Geometry check sheet. Reference: the model listing, model coordinates, mm. Give positions to 0.01 mm unless a question says otherwise; leave off trailing zeros. Loops run counter-clockwise (first coordinate to the right, second up) from the corner with the lowest first, then second, coordinate; pieces in that order, holes last. Notation, with made-up numbers: (29, -33) -> (47, -33) arc R10 ccw to (47, -28) -> close; hole circle Ø5 at (23.25, 85). An arc over 180 degrees is marked (long way). Answer in a Markdown table with one row per item. Add a question column.
Autodesk Inventor part; units mm, degrees
ref_plane "YZ Plane" through (0, 0, 0) normal (1, 0, 0) x (0, 1, 0)
ref_plane "XZ Plane" through (0, 0, 0) normal (0, 1, 0) x (-1, 0, 0)
ref_plane "XY Plane" through (0, 0, 0) normal (0, 0, 1) x (1, 0, 0)
sketch "Sketch1" plane through (0, 0, 0) normal (0, 1, 0) x (-1, 0, 0)
  circle A0 centre (0, 0) radius 73.025
  circle A1 centre (0, 0) radius 84.1375
  line L0 (0, 0) -> (0, 84.1375) construction
  circle A2 centre (0, 65.0875) radius 1.7526
  circle A3 centre (0, 65.0875) radius 7.9375 construction
  circle A4 centre (-61.9019, 20.1131) radius 1.7526
  circle A5 centre (-61.9019, 20.1131) radius 7.9375 construction
  circle A6 centre (-38.2575, -52.6569) radius 1.7526
  circle A7 centre (-38.2575, -52.6569) radius 7.9375 construction
  circle A8 centre (38.2575, -52.6569) radius 1.7526
  circle A9 centre (38.2575, -52.6569) radius 7.9375 construction
  circle A10 centre (61.9019, 20.1131) radius 1.7526
  circle A11 centre (61.9019, 20.1131) radius 7.9375 construction
  arc A12 (-29.3651, -56.0703) -> (-44.2517, -45.2546) centre (-38.2575, -52.6569) ccw
  line L1 (-29.3651, -56.0703) -> (-32.8726, -65.2077)
  line L2 (-44.2517, -45.2546) -> (-51.858, -51.414)
  arc A13 (44.2517, -45.2546) -> (29.3651, -56.0703) centre (38.2575, -52.6569) ccw
  line L3 (29.3651, -56.0703) -> (32.8726, -65.2077)
  line L4 (44.2517, -45.2546) -> (51.858, -51.414)
  arc A14 (-5.2592, 57.1461) -> (5.2592, 57.1461) centre (0, 65.0875) ccw
  arc A15 (55.1667, 26.8483) -> (61.9019, 10.5881) centre (61.9019, 20.1131) ccw
  line L5 (61.9019, 10.5881) -> (72.2533, 10.5881)
  line L6 (0, 0) -> (61.9019, 20.1131) construction
  line L7 (55.1667, 26.8483) -> (63.8164, 35.4981)
  arc A16 (-61.9019, 10.5881) -> (-55.1667, 26.8483) centre (-61.9019, 20.1131) ccw
  line L8 (-61.9019, 10.5881) -> (-72.2533, 10.5881)
  line L9 (-55.1667, 26.8483) -> (-63.8164, 35.4981)
  line L10 (0, 0) -> (12.6807, 71.9156) construction
  circle A17 centre (11.8537, 67.2254) radius 3.3655
  circle A18 centre (0, 0) radius 68.2625 construction
  circle A19 centre (11.8537, 67.2254) radius 4.7625 construction
  circle A20 centre (-11.8537, 67.2254) radius 3.3655
  circle A21 centre (-11.8537, 67.2254) radius 4.7625 construction
  line L11 (-5.2592, 57.1461) -> (-23.4145, 69.1694)
  line L12 (5.2592, 57.1461) -> (23.4145, 69.1694)
  line L13 (7.9375, -79.375) -> (-7.9375, -79.375)
  line L14 (-7.9375, -79.375) -> (-7.9375, -73.025)
  line L15 (-7.9375, -73.025) -> (7.9375, -73.025)
  line L16 (7.9375, -73.025) -> (7.9375, -79.375)
  line L17 (7.9375, -79.375) -> (-7.9375, -73.025) construction
  line L18 (-7.9375, -79.375) -> (7.9375, -73.025) construction
  line L19 (0, -76.2) -> (0, -84.1375) construction
  line L20 (12.7, -82.55) -> (-12.7, -82.55) construction
  line L21 (-12.7, -82.55) -> (-12.7, -69.85)
  line L22 (-12.7, -69.85) -> (12.7, -69.85)
  line L23 (12.7, -69.85) -> (12.7, -82.55)
  line L24 (12.7, -82.55) -> (-12.7, -69.85) construction
  line L25 (-12.7, -82.55) -> (12.7, -69.85) construction
  line L26 (30.7823, -63.9747) -> (51.3313, -49.045)
  line L27 (36.5014, -63.744) -> (49.3446, -54.4129)
  line L28 (53.077, -59.5502) -> (40.2339, -68.8813)
  line L29 (40.2339, -68.8813) -> (36.5014, -63.744)
  line L30 (49.3446, -54.4129) -> (53.077, -59.5502)
  line L31 (53.077, -59.5502) -> (36.5014, -63.744) construction
  line L32 (40.2339, -68.8813) -> (49.3446, -54.4129) construction
  line L33 (51.3313, -49.045) -> (58.7962, -59.3195)
  line L34 (58.7962, -59.3195) -> (38.2472, -74.2492) construction
  line L35 (38.2472, -74.2492) -> (51.3313, -49.045) construction
  line L36 (58.7962, -59.3195) -> (30.7823, -63.9747) construction
  line L37 (38.2472, -74.2492) -> (30.7823, -63.9747)
  line L38 (62.5068, -33.6633) -> (70.3558, -9.5064)
  line L39 (66.9981, -30.115) -> (71.9037, -15.017)
  line L40 (77.9429, -16.9792) -> (73.0373, -32.0772)
  line L41 (73.0373, -32.0772) -> (66.9981, -30.115)
  line L42 (71.9037, -15.017) -> (77.9429, -16.9792)
  line L43 (77.9429, -16.9792) -> (66.9981, -30.115) construction
  line L44 (73.0373, -32.0772) -> (71.9037, -15.017) construction
  line L45 (70.3558, -9.5064) -> (82.4342, -13.4309)
  line L46 (82.4342, -13.4309) -> (74.5852, -37.5878) construction
  line L47 (74.5852, -37.5878) -> (70.3558, -9.5064) construction
  line L48 (82.4342, -13.4309) -> (62.5068, -33.6633) construction
  line L49 (74.5852, -37.5878) -> (62.5068, -33.6633)
  line L50 (70.3558, 9.5064) -> (62.5068, 33.6633)
  line L51 (71.9037, 15.017) -> (66.9981, 30.115)
  line L52 (73.0373, 32.0772) -> (77.9429, 16.9792)
  line L53 (77.9429, 16.9792) -> (71.9037, 15.017)
  line L54 (66.9981, 30.115) -> (73.0373, 32.0772)
  line L55 (73.0373, 32.0772) -> (71.9037, 15.017) construction
  line L56 (77.9429, 16.9792) -> (66.9981, 30.115) construction
  line L57 (62.5068, 33.6633) -> (74.5852, 37.5878)
  line L58 (74.5852, 37.5878) -> (82.4342, 13.4309) construction
  line L59 (82.4342, 13.4309) -> (62.5068, 33.6633) construction
  line L60 (74.5852, 37.5878) -> (70.3558, 9.5064) construction
  line L61 (82.4342, 13.4309) -> (70.3558, 9.5064)
  line L62 (51.3313, 49.045) -> (30.7823, 63.9747)
  line L63 (49.3446, 54.4129) -> (36.5014, 63.744)
  line L64 (40.2339, 68.8813) -> (53.077, 59.5502)
  line L65 (53.077, 59.5502) -> (49.3446, 54.4129)
  line L66 (36.5014, 63.744) -> (40.2339, 68.8813)
  line L67 (40.2339, 68.8813) -> (49.3446, 54.4129) construction
  line L68 (53.077, 59.5502) -> (36.5014, 63.744) construction
  line L69 (30.7823, 63.9747) -> (38.2472, 74.2492)
  line L70 (38.2472, 74.2492) -> (58.7962, 59.3195) construction
  line L71 (58.7962, 59.3195) -> (30.7823, 63.9747) construction
  line L72 (38.2472, 74.2492) -> (51.3313, 49.045) construction
  line L73 (58.7962, 59.3195) -> (51.3313, 49.045)
  circle A22 centre (0, 0) radius 69.85
  line L74 (17.6671, 70.8557) -> (16.0268, 64.2769)
  line L75 (-17.6671, 70.8557) -> (-16.0268, 64.2769)
  line L76 (-38.2575, -52.6569) -> (-49.4548, -68.0687) construction
  line L77 (12.7, 69.85) -> (-12.7, 69.85)
  line L78 (7.9375, 73.025) -> (-7.9375, 73.025)
  line L79 (-7.9375, 79.375) -> (7.9375, 79.375)
  line L80 (7.9375, 79.375) -> (7.9375, 73.025)
  line L81 (-7.9375, 73.025) -> (-7.9375, 79.375)
  line L82 (-7.9375, 79.375) -> (7.9375, 73.025) construction
  line L83 (7.9375, 79.375) -> (-7.9375, 73.025) construction
  line L84 (-12.7, 69.85) -> (-12.7, 82.55)
  line L85 (-12.7, 82.55) -> (12.7, 82.55) construction
  line L86 (12.7, 82.55) -> (-12.7, 69.85) construction
  line L87 (-12.7, 82.55) -> (12.7, 69.85) construction
  line L88 (12.7, 82.55) -> (12.7, 69.85)
  line L89 (-30.7823, 63.9747) -> (-51.3313, 49.045)
  line L90 (-36.5014, 63.744) -> (-49.3446, 54.4129)
  line L91 (-53.077, 59.5502) -> (-40.2339, 68.8813)
  line L92 (-40.2339, 68.8813) -> (-36.5014, 63.744)
  line L93 (-49.3446, 54.4129) -> (-53.077, 59.5502)
  line L94 (-53.077, 59.5502) -> (-36.5014, 63.744) construction
  line L95 (-40.2339, 68.8813) -> (-49.3446, 54.4129) construction
  line L96 (-51.3313, 49.045) -> (-58.7962, 59.3195)
  line L97 (-58.7962, 59.3195) -> (-38.2472, 74.2492) construction
  line L98 (-38.2472, 74.2492) -> (-51.3313, 49.045) construction
  line L99 (-58.7962, 59.3195) -> (-30.7823, 63.9747) construction
  line L100 (-38.2472, 74.2492) -> (-30.7823, 63.9747)
  line L101 (-62.5068, 33.6633) -> (-70.3558, 9.5064)
  line L102 (-66.9981, 30.115) -> (-71.9037, 15.017)
  line L103 (-77.9429, 16.9792) -> (-73.0373, 32.0772)
  line L104 (-73.0373, 32.0772) -> (-66.9981, 30.115)
  line L105 (-71.9037, 15.017) -> (-77.9429, 16.9792)
  line L106 (-77.9429, 16.9792) -> (-66.9981, 30.115) construction
  line L107 (-73.0373, 32.0772) -> (-71.9037, 15.017) construction
  line L108 (-70.3558, 9.5064) -> (-82.4342, 13.4309)
  line L109 (-82.4342, 13.4309) -> (-74.5852, 37.5878) construction
  line L110 (-74.5852, 37.5878) -> (-70.3558, 9.5064) construction
  line L111 (-82.4342, 13.4309) -> (-62.5068, 33.6633) construction
  line L112 (-74.5852, 37.5878) -> (-62.5068, 33.6633)
  line L113 (-70.3558, -9.5064) -> (-62.5068, -33.6633)
  line L114 (-71.9037, -15.017) -> (-66.9981, -30.115)
  line L115 (-73.0373, -32.0772) -> (-77.9429, -16.9792)
  line L116 (-77.9429, -16.9792) -> (-71.9037, -15.017)
  line L117 (-66.9981, -30.115) -> (-73.0373, -32.0772)
  line L118 (-73.0373, -32.0772) -> (-71.9037, -15.017) construction
  line L119 (-77.9429, -16.9792) -> (-66.9981, -30.115) construction
  line L120 (-62.5068, -33.6633) -> (-74.5852, -37.5878)
  line L121 (-74.5852, -37.5878) -> (-82.4342, -13.4309) construction
  line L122 (-82.4342, -13.4309) -> (-62.5068, -33.6633) construction
  line L123 (-74.5852, -37.5878) -> (-70.3558, -9.5064) construction
  line L124 (-82.4342, -13.4309) -> (-70.3558, -9.5064)
  line L125 (-51.3313, -49.045) -> (-30.7823, -63.9747)
  line L126 (-49.3446, -54.4129) -> (-36.5014, -63.744)
  line L127 (-40.2339, -68.8813) -> (-53.077, -59.5502)
  line L128 (-53.077, -59.5502) -> (-49.3446, -54.4129)
  line L129 (-36.5014, -63.744) -> (-40.2339, -68.8813)
  line L130 (-40.2339, -68.8813) -> (-49.3446, -54.4129) construction
  line L131 (-53.077, -59.5502) -> (-36.5014, -63.744) construction
  line L132 (-30.7823, -63.9747) -> (-38.2472, -74.2492)
  line L133 (-38.2472, -74.2492) -> (-58.7962, -59.3195) construction
  line L134 (-58.7962, -59.3195) -> (-30.7823, -63.9747) construction
  line L135 (-38.2472, -74.2492) -> (-51.3313, -49.045) construction
  line L136 (-58.7962, -59.3195) -> (-51.3313, -49.045)
  line L137 (7.633, 69.4317) -> (8.401, 59.2267)
  line L138 (-7.633, 69.4317) -> (-8.401, 59.2267)
  point P0 (51.858, -51.414)
  point P1 (64.5887, 34.0727)
  point P2 (44.7892, -61.6471)
  point P3 (72.4705, -23.5471)
  point P4 (72.4705, 23.5471)
  point P5 (44.7892, 61.6471)
  point P6 (12.7, -71.9122)
  point P7 (-12.7, -71.9122)
  point P8 (31.9944, 65.643)
  point P9 (52.5434, 50.7133)
  point P10 (64.468, 34.3005)
  point P11 (72.3171, 10.1437)
  point P12 (72.3171, -10.1437)
  point P13 (64.468, -34.3005)
  point P14 (52.5434, -50.7133)
  point P15 (31.9944, -65.643)
  point P16 (66.4313, 21.5848)
  point P17 (-20.018, 66.9201)
  point P18 (-61.4776, 33.1592)
  point P19 (20.018, 66.9201)
  point P20 (66.4313, -21.5848)
  point P21 (61.4776, 33.1592)
  point P22 (41.0568, -56.5098)
  point P23 (69.0428, 10.5881)
  point P24 (49.3775, -49.4053)
  point P25 (41.0568, 56.5098)
  point P26 (-69.0428, 10.5881)
  point P27 (-49.3775, -49.4053)
  point P28 (31.7288, -62.2279)
  point P29 (0, -69.85)
  point P30 (-31.7288, -62.2279)
  point P31 (0, 76.2)
  point P32 (-44.7892, 61.6471)
  point P33 (-72.4705, 23.5471)
  point P34 (-72.4705, -23.5471)
  point P35 (-44.7892, -61.6471)
  point P36 (32.0467, -63.0561)
  point P37 (50.0669, -49.9636)
  point P38 (70.0043, 10.5881)
  point P39 (62.7968, 32.7708)
  point P40 (12.7, 71.9122)
  point P41 (12.7, 70.4828)
  point P42 (9.1625, 69.2464)
  point P43 (-9.1625, 69.2464)
  point P44 (-12.7, 70.4828)
  point P45 (-12.7, 71.9122)
  point P46 (16.899, 67.775)
  point P47 (15.0737, 68.2041)
  point P48 (-15.0737, 68.2041)
  point P49 (-16.899, 67.775)
  dimension "d1" = 146.05
  dimension "d13" = 136.525
  dimension "d14" = 9.525
  dimension "d78" = 3.175
  dimension "d0" = 11.1125
  dimension "d2" = 3.5052
  dimension "d3" = 15.875
  dimension "d6" = 360
  dimension "d8" = 19.05
  dimension "d9" = 19.05
  dimension "d10" = 19.05
  dimension "d11" = 10
  dimension "d12" = 6.731
  dimension "d34" = 15.875
  dimension "d35" = 6.35
  dimension "d37" = 25.4
  dimension "d39" = 3.175
  dimension "d42" = 360
  dimension "d151" = 76.2
  dimension "d153" = 15
  dimension "d163" = 90
extrude "Extrusion1" add sketch "Sketch1" along normal blind 9.525 contours L12 A14 L11 L138 A22 L137
fillet "Fillet14" radius 3.175 4 edges at (-7.633, 4.7625, 69.4317) (-8.401, 4.7625, 59.2267) (8.401, 4.7625, 59.2267) (7.633, 4.7625, 69.4317)
chamfer "Chamfer15" distance 3.175 angle 45 1 edges at (1.7526, 9.525, 65.0875)
equation "\"d1\" = Ring_ID"
equation "\"BearingTol\" = 0.1"
equation "\"CSDepth\" = 1.7272"
equation "\"CSAngle\" = 41deg"
properties part number "Retaining Ring" material "UHMW, White"
1. Sectioned sample at C-C (x = 5.75). Enter the section's corners in (y, z) (3 decimals), plus the area to 3 significant figures.
2. Material ranges on L1, parallel to Z at x = 0, y = 1.75; L2, parallel to Z at x = 0.5, y = 8.75; L3, parallel to X at y = 4, z = 66.5, recorded low to high. Write a range as from..to.
3. Release check for a two-part mould opening along Z. For faces 1 (the face through (0.254, 6.549, 67.022)), 2 (the face through (0, 0, 63)), 3 (the face through (-6.043, 4.696, 57.665)) record: released by +Z, released by -Z, zero draft, split by the parting line, or undercut.
4. Sectioned sample at D-D (x = -5.5). Enter the section's corners in (y, z) (3 decimals), plus the area to 3 significant figures.
5. Sectioned sample at A-A (x = 0). Enter the section's corners in (y, z) (3 decimals).
6. Gauge pin test, flat ends, axial feed: pin 1 Ø1 at (x, y) = (-6, 5.5) entering from -Z; pin 2 Ø2 at (x, y) = (-3, 4) entering from -Z; pin 3 Ø1.5 at (x, z) = (3, 66.5) entering from +Y. Record the tip position at first contact, or that the pin passes through.
Response:
| question | item | result |
|---|---|---|
| 1 | outline | (0, 57.471) -> (9.525, 57.471) -> (9.525, 69.497) -> (0, 69.497) -> close |
| 1 | area | 115 mm2 |
| 2 | L1 | z = 55.56..63.33, 66.84..69.85 |
| 2 | L2 | z = 55.58..60.97, 69.21..69.85 |
| 2 | L3 | x = -7.85..-1.04, 1.04..7.85 |
| 3 | face 1 | undercut |
| 3 | face 2 | zero draft |
| 3 | face 3 | released by -Z |
| 4 | outline | (0, 57.306) -> (9.525, 57.306) -> (9.525, 69.576) -> (0, 69.576) -> close |
| 4 | area | 117 mm2 |
| 5 | outline | (0, 55.563) -> (9.525, 55.563) -> (9.525, 60.16) -> (6.35, 63.335) -> (0, 63.335) -> close; (0, 66.84) -> (6.35, 66.84) -> (9.36, 69.85) -> (0, 69.85) -> close |
| 6 | pin 1 | stops at z = 57.31 |
| 6 | pin 2 | stops at z = 55.77 |
| 6 | pin 3 | stops at y = 8.66 |
